Build history of the part. All positions in model axes, mm. A direction names the side the tool comes from. Round coordinates to 2 decimals unless told otherwise and drop trailing zeros. Order: outer loops, then holes, each group sorted by start corner. A loop starts at its lowest first (then second) coordinate and runs counter-clockwise, first axis right, second up. Notation, with made-up numbers: M -10,-22 L 31,-22 A23 cw 31,12 Z; hole C 57,57.25 d1. An arc over 180 degrees is marked long. One line per item, written item: value. Start each with the question number.
Item 1: Pin check, flat tips, straight feed: pin 1 (2 mm diameter, centred on y = 16.5, z = 2, fed in from -X); pin 2 (2 mm diameter, centred on x = 20.5, y = 37, fed in from +Z) (3 decimals). Stop position of each tip, or through.
Item 2: Band-saw the part on A-A, the plane z = 2.5. Write the cut outline in (x, y), then the cut area to 3 significant figures.
Item 3: Band-saw the part on C-C, the plane y = 49.5. Write the cut outline in (x, z) (3 decimals), then the cut area to 4 significant figures.
Item 4: Tool access for faces 1 (the flat face through (-1, 48, 3)), 2 (the flat face through (0, 54, 2)), 3 (the flat face through (14, 56, 2)): list every direction of +Z, -Z, +X, -X, +Y, -Y with a clear straight run to the whole face (end or side of a thin tool).
Item 5: Probe L1, parallel to X at y = 40, z = 0.7; L2, parallel to X at y = 48.5, z = 1.15; L3, parallel to Y at x = 20, z = 2.3. List the from-to ranges inside material, lowest first.
Item 6: Two-plate mould, pull along Y, no slides. Class faces 4 (the flat face through (14, 0, 2)), 5 (the flat face through (-1.1, 51.1, 2)), 6 (the flat face through (0, 50.5, 2)): +Y half, -Y half, draft (parallel to the pull), parting line (faces both ways), or undercut.
Item 7: Band-saw the part on D-D, the plane y = 5. Write the cut outline in (x, z) (3 decimals).
Item 8: Band-saw the part on B-B, the plane x = 21.5. Write the cut outline in (y, z) (3 decimals).
```python
from build123d import *

# Parameters (mm, degrees)
BOX_W           = 28
BOX_H           = 56
BOX_DEPTH       = 0.125
SKETCH004_W     = 1.5
SKETCH004_H     = 45.5
SKETCH004_H_2   = 4
PAD004_DEPTH    = 4
SKETCH005_W     = 28
SKETCH005_H     = 1.5
PAD005_DEPTH    = 4
SKETCH006_W     = 1.5
SKETCH006_H     = 53
PAD006_DEPTH    = 4
SKETCH003_W     = 28
SKETCH003_H     = 1.5
PAD003_DEPTH    = 4
BOX004_W        = 5
BOX004_H        = 5
BOX004_DEPTH    = 5
CHAMFER_SIZE    = 1
BOX002_W        = 2
BOX002_H        = 8
BOX002_DEPTH    = 4.125
CHAMFER001_SIZE = 1.8


with BuildPart() as base:
    # Box → Box (new body)
    with BuildSketch(Plane.XY):
        with Locations((14, 28)):
            Rectangle(BOX_W, BOX_H)
    extrude(amount=BOX_DEPTH)


with BuildPart() as pad004:
    # Sketch004 → Pad004 (new body)
    with BuildSketch(Plane.XY.offset(0.125)):
        with Locations((0.75, 22.75)):
            Rectangle(SKETCH004_W, SKETCH004_H)
        with Locations((0.75, 52.5)):
            Rectangle(SKETCH004_W, SKETCH004_H_2)
    extrude(amount=PAD004_DEPTH)


with BuildPart() as pad005:
    # Sketch005 → Pad005 (new body)
    with BuildSketch(Plane.XY.offset(0.125)):
        with Locations((14, 0.75)):
            Rectangle(SKETCH005_W, SKETCH005_H)
    extrude(amount=PAD005_DEPTH)


with BuildPart() as pad006:
    # Sketch006 → Pad006 (new body)
    with BuildSketch(Plane.XY.offset(0.125)):
        with Locations((27.25, 28)):
            Rectangle(SKETCH006_W, SKETCH006_H)
    extrude(amount=PAD006_DEPTH)


with BuildPart() as walls:
    # Sketch003 → Pad003 (new body)
    with BuildSketch(Plane.XY.offset(0.125)):
        with Locations((14, 55.25)):
            Rectangle(SKETCH003_W, SKETCH003_H)
    extrude(amount=PAD003_DEPTH)

    # Fusion001: union Pad004, Pad005, Pad006
    add(pad004.part)
    add(pad005.part)
    add(pad006.part)


with BuildPart() as chamfer_body:
    # Box004 → Box004 (new body)
    with BuildSketch(Plane(origin=(-1, 45.5, 0.125), x_dir=(1, 0, 0), z_dir=(0, 0, 1))):
        with Locations((2.5, 2.5)):
            Rectangle(BOX004_W, BOX004_H)
    extrude(amount=BOX004_DEPTH)

    # Chamfer
    chamfer_edges = [chamfer_body.edges().sort_by_distance(p)[0] for p in [
        (-1, 48, 0.125),
    ]]
    chamfer(chamfer_edges, length=CHAMFER_SIZE)


with BuildPart() as base_and_walls_do_not_edit:
    # Box002 → Box002 (new body)
    with BuildSketch(Plane(origin=(-2, 44, 0), x_dir=(1, 0, 0), z_dir=(0, 0, 1))):
        with Locations((1, 4)):
            Rectangle(BOX002_W, BOX002_H)
    extrude(amount=BOX002_DEPTH)

    # Chamfer001
    chamfer001_edges = [base_and_walls_do_not_edit.edges().sort_by_distance(p)[0] for p in [
        (-2, 44, 2.0625),
        (-2, 52, 2.0625),
    ]]
    chamfer(chamfer001_edges, length=CHAMFER001_SIZE)

    # Cut: cut Chamfer body
    add(chamfer_body.part, mode=Mode.SUBTRACT)

    # Fusion: union Walls
    add(walls.part)

    # Fusion002: union Base
    add(base.part)


solid = base_and_walls_do_not_edit.part
```
Output:
1. pin 1: stops at x = 0
1. pin 2: stops at z = 0.125
2. outline: M -2,45.8 L -0.2,44 L 0,44 L 0,0 L 28,0 L 28,56 L 0,56 L 0,52 L -0.2,52 L -2,50.2 Z; hole M -1,45.5 L 1.5,45.5 L 1.5,1.5 L 26.5,1.5 L 26.5,54.5 L 1.5,54.5 L 1.5,50.5 L -1,50.5 Z
2. area: 243 mm²
3. outline: M -2,0 L 28,0 L 28,4.125 L 26.5,4.125 L 26.5,0.125 L 0,0.125 L -1,1.125 L -1,4.125 L -2,4.125 Z
3. area: 14.25 mm²
4. face 1: +Z
4. face 2: +Z, -Z, -X, +Y
4. face 3: +Z, -Z, +X, -X, +Y
5. L1: x = 0 to 1.5, 26.5 to 28
5. L2: x = -2 to -1, 26.5 to 28
5. L3: y = 0 to 1.5, 54.5 to 56
6. face 4: -Y half
6. face 5: +Y half
6. face 6: undercut
7. outline: M 0,0 L 28,0 L 28,4.125 L 26.5,4.125 L 26.5,0.125 L 1.5,0.125 L 1.5,4.125 L 0,4.125 Z
8. outline: M 0,0 L 56,0 L 56,4.125 L 54.5,4.125 L 54.5,0.125 L 1.5,0.125 L 1.5,4.125 L 0,4.125 Z
